from build123d import *

# Parameters (mm, degrees)
BOSS_EXTRUDE2_DEPTH     = 20
FILLET1_R               = 10
CUT_EXTRUDE2_REACH      = 31.799
CUT_EXTRUDE2_END_RADIUS = 16.5
SKETCH4_R               = 2.8408
CUT_EXTRUDE3_START      = -2.5
SKETCH5_R               = 3.21845
CUT_EXTRUDE3_DEPTH      = 1.38
BOSS_EXTRUDE3_START     = -6
SKETCH6_R               = 1.75
BOSS_EXTRUDE3_DEPTH     = 4


with BuildPart() as part:
    # Sketch3 → Boss-Extrude2 (new body)
    with BuildSketch(Plane(origin=(0, 0, 0), x_dir=(0, 0, -1), z_dir=(1, 0, 0))):
        with BuildLine():
            Line((0, 20), (-9.38, 20))
            Line((-9.38, 20), (-9.38, 0))
            Line((-9.38, 0), (0, 0))
            ThreePointArc((0, 0), (-3.375595252, 10), (0, 20))
        make_face()
    extrude(amount=BOSS_EXTRUDE2_DEPTH)

    # Fillet1
    fillet1_edges = [part.edges().sort_by_distance(p)[0] for p in [
        (20, 0, 4.69),
        (0, 0, 4.69),
        (20, 20, 4.69),
        (0, 20, 4.69),
    ]]
    fillet(fillet1_edges, radius=FILLET1_R - 0.0001)  # a hair under: the kernel refuses the full size

    # Cut-Extrude2: up to this cylinder (the profile starts outside it)
    cut_extrude2_end = Plane(origin=(10, 10, -13.124404748), z_dir=(-1, 0, 0)) * Cylinder(CUT_EXTRUDE2_END_RADIUS, 97.598, mode=Mode.PRIVATE)
    # Sketch4 → Cut-Extrude2 (cut, up to the surface)
    with BuildSketch(Plane.XY.offset(9.38), mode=Mode.PRIVATE) as cut_extrude2_sk1:
        with Locations((10, 10)):
            Circle(SKETCH4_R)
    cut_extrude2_tool1 = extrude(cut_extrude2_sk1.sketch, amount=-CUT_EXTRUDE2_REACH, mode=Mode.PRIVATE) - cut_extrude2_end
    add(cut_extrude2_tool1.solids().sort_by_distance((10, 10, 9.38))[0], mode=Mode.SUBTRACT)

    # Sketch5 → Cut-Extrude3 (cut)
    with BuildSketch(Plane.XY.offset(9.38).offset(CUT_EXTRUDE3_START)):
        with Locations((10, 10)):
            Circle(SKETCH5_R)
    extrude(amount=-CUT_EXTRUDE3_DEPTH, mode=Mode.SUBTRACT)

    # Sketch6 → Boss-Extrude3 (add)
    with BuildSketch(Plane.XY.offset(9.38).offset(BOSS_EXTRUDE3_START)):
        with Locations((3.5, 10)):
            Circle(SKETCH6_R)
        with Locations((16.5, 10)):
            Circle(SKETCH6_R)
    extrude(amount=-BOSS_EXTRUDE3_DEPTH)


solid = part.part
Input: part model. Units: mm. Frame: model coordinates. A direction names the side the tool comes from. Give positions to 0.01 mm unless a question says otherwise; leave off trailing zeros. Write each loop counter-clockwise with the first axis right and the second up, starting at its lowest first coordinate (ties: lowest second). Pieces come first, ordered by that corner, then holes. Notation, with made-up numbers: M -27,65.5 L 10,65.5 A7 cw 10,75.5 Z; hole C 34,55 d9. An arc over 180 degrees is marked long. Write item = value, one per line. Start each with the question number.
1) Cut plane A-A on z = 0.5. Count the separate pieces of the cut face and the enclosed holes in it, then the cut area to 3 significant figures.
2) Reachability of faces 1 (the cylindrical face through (12.71, 10.85, 8.15)), 2 (the cylindrical face through (3.272, 11.735, 1.407)), 3 (the flat face through (10, 7, 5.5)) from +Z, -Z, +X, -X, +Y, -Y: full face, straight path, thin tool, end or side. Return the list, or none.
3) Cut plane D-D on x = 3.5. Return the cut outline in (y, z).
4) Material intervals for line 1 along Y through (x, z) = (10, 4.5); line 2 along Y through (x, z) = (10, 6.15), sorted ascending. Write a range as [from, to].
5) First-contact query: pin 1 Ø2 at (y, z) = (7.5, 5.5) entering from -X; pin 2 Ø6.5 at (x, y) = (10, 10) entering from +Z; pin 3 Ø1.5 at (x, y) = (7.5, 10) entering from -Z. Flat tips, straight axial feed; report the tip coordinate or a pass-through.
6) Cut plane B-B on y = 10.75. Return the cut outline in (x, z).
7) Draft query along Y for faces 4 (the cylindrical face through (3.01, 17.15, 5.8)), 5 (the cylindrical face through (16.99, 2.85, 5.67)), 6 (the flat face through (16, 10, -0.62)), 7 (the cylindrical face through (11.485, 7.145, 6.2)). Return one class per face: +Y half, -Y half, draft (parallel to the pull), parting line (faces both ways), or undercut.
Solved:
q1.separate_pieces = 4
q1.enclosed_holes = 0
q1.area = 26.0 mm2
q2.face_1 = +Z, -Z
q2.face_2 = -Z
q2.face_3 = none
q3.outline = M 2.4,1.52 A16.5 cw 8.25,3.28 L 8.25,-0.62 L 11.75,-0.62 L 11.75,3.28 A16.5 cw 17.6,1.52 L 17.6,9.38 L 2.4,9.38 Z
q4.line_1 = [0, 7.16], [12.84, 20]
q4.line_2 = [0, 6.78], [13.22, 20]
q5.pin_1 = 0.11
q5.pin_2 = 9.38
q5.pin_3 = 3.36
q6.outline = M 0.03,3.36 L 1.92,3.36 L 1.92,-0.62 L 5.08,-0.62 L 5.08,3.36 L 7.26,3.36 L 7.26,5.5 L 6.87,5.5 L 6.87,6.88 L 7.26,6.88 L 7.26,9.38 L 0.03,9.38 Z; M 12.74,3.36 L 14.92,3.36 L 14.92,-0.62 L 18.08,-0.62 L 18.08,3.36 L 19.97,3.36 L 19.97,9.38 L 12.74,9.38 L 12.74,6.88 L 13.13,6.88 L 13.13,5.5 L 12.74,5.5 Z
q7.face_4 = +Y half
q7.face_5 = -Y half
q7.face_6 = draft
q7.face_7 = undercut
